```python
from build123d import *

# Parameters (mm, degrees)
SKETCH1_W              = 40
SKETCH1_H              = 60
BOSS_EXTRUDE1_DEPTH    = 10
M2_5_CLEARANCE_HOLE1_D = 2.9
CUT_EXTRUDE1_DEPTH     = 6.2
FILLET1_R              = 1.6
CHAMFER1_SIZE          = 1


with BuildPart() as part:
    # Sketch1 → Boss-Extrude1 (new body)
    with BuildSketch(Plane(origin=(0, 0, 0), x_dir=(1, 0, 0), z_dir=(0, 1, 0))):
        with Locations((-20, 0)):
            Rectangle(SKETCH1_W, SKETCH1_H)
    extrude(amount=BOSS_EXTRUDE1_DEPTH)

    # M2.5 Clearance Hole1 (through all)
    with Locations(Plane(origin=(0, 10, 0), x_dir=(1, 0, 0), z_dir=(0, 1, 0))):
        with Locations((-37.3, 26), (-37.3, 4), (-37.3, -18), (-31, -25.8), (-9, -25.8), (-2.7, -18), (-2.7, 4), (-2.7, 26)):
            Hole(M2_5_CLEARANCE_HOLE1_D / 2)

    # Sketch4 → Cut-Extrude1 (cut)
    with BuildSketch(Plane(origin=(0, 10, 0), x_dir=(1, 0, 0), z_dir=(0, 1, 0))):
        Polygon((-34.6, 30), (-34.6, -19), (-30, -19), (-30, -23), (-10, -23), (-10, -19), (-5.4, -19), (-5.4, 30), align=None)
    extrude(amount=-CUT_EXTRUDE1_DEPTH, mode=Mode.SUBTRACT)

    # Fillet1
    fillet1_edges = [part.edges().sort_by_distance(p)[0] for p in [
        (-10, 6.9, 23),
        (-30, 6.9, 23),
        (-30, 6.9, 19),
        (-34.6, 6.9, 19),
        (-5.4, 6.9, 19),
        (-10, 6.9, 19),
    ]]
    fillet(fillet1_edges, radius=FILLET1_R)

    # Chamfer1
    chamfer1_edges = [part.edges().sort_by_distance(p)[0] for p in [
        (-40, 5, -30),
        (0, 5, -30),
        (0, 5, 30),
        (-40, 5, 30),
    ]]
    chamfer(chamfer1_edges, length=CHAMFER1_SIZE)


solid = part.part
```
Geometry check sheet. Reference: the model listing, model coordinates, mm. A direction names the side the tool comes from. Round coordinates to 2 decimals unless told otherwise and drop trailing zeros. Order: outer loops, then holes, each group sorted by start corner. A loop starts at its lowest first (then second) coordinate and runs counter-clockwise, first axis right, second up. Notation, with made-up numbers: (-25.75, -38.75) - (-18.75, -38.75) arc R32 ccw to (-18.75, 0.25) - close; hole circle Ø11 at (-18.75, -4). An arc over 180 degrees is marked (long way). Use a Markdown table: item, result. Add a question column.
1) Mould release check, pull along X, two halves, no side actions. Record for faces 1 (the flat face through (-40, 5, 0)), 2 (the cylindrical face through (-7.93, 4.93, 24.82)), 3 (the cylindrical face through (-2.386, 4.93, 19.416)), 4 (the flat face through (-35, 10, 9)): released by +X, released by -X, zero draft, split by the parting line, or undercut.
2) Set-up check for faces 5 (the cylindrical face through (-30.48, 6.86, 19.46)), 6 (the cylindrical face through (-36.15, 4.93, -25.12)): record each of +Z, -Z, +X, -X, +Y, -Y from which the full face is reachable in a straight line by a thin tool's end or side.
3) Section check B-B (z = 25.8). Record the cut outline in (x, y), then the cut area to 3 significant figures.
4) Section check A-A (x = -2.7). Record the cut outline in (y, z), then the cut area to 3 significant figures.
5) Gauge pin test, flat ends, axial feed: P1, Ø6, axis at x = -25.5, z = -10, coming from the +Y side; P2, Ø5, axis at x = -18.5, y = 8.5, coming from the -Z side. Record the tip position at first contact, or that the pin passes through.
6) Section check C-C (y = 2). Count the separate pieces of the cut face and the enclosed holes in it, then the cut area to 3 significant figures.
7) Thickness scan on line 1 along Z through (x, y) = (-2.7, 3.5); line 2 along X through (y, z) = (6.25, 25.8); line 3 along X through (y, z) = (2.25, -26). Record the ranges inside material, lowest first.
Established:
| question | item | result |
|---|---|---|
| 1 | face 1 | released by -X |
| 1 | face 2 | undercut |
| 1 | face 3 | undercut |
| 1 | face 4 | zero draft |
| 2 | face 5 | -Z, +Y |
| 2 | face 6 | +Y, -Y |
| 3 | outline | (-40, 0) - (-32.45, 0) - (-32.45, 10) - (-40, 10) - close; (-29.55, 0) - (-10.45, 0) - (-10.45, 10) - (-29.55, 10) - close; (-7.55, 0) - (0, 0) - (0, 10) - (-7.55, 10) - close |
| 3 | area | 342 mm2 |
| 4 | outline | (0, -30) - (10, -30) - (10, -27.45) - (0, -27.45) - close; (0, -24.55) - (10, -24.55) - (10, -5.45) - (0, -5.45) - close; (0, -2.55) - (10, -2.55) - (10, 16.55) - (0, 16.55) - close; (0, 19.45) - (10, 19.45) - (10, 30) - (0, 30) - close |
| 4 | area | 513 mm2 |
| 5 | P1 | y = 3.8 |
| 5 | P2 | z = 23 |
| 6 | separate pieces | 1 |
| 6 | enclosed holes | 8 |
| 6 | area | 2,350 mm2 |
| 7 | line 1 | -30 to -27.45, -24.55 to -5.45, -2.55 to 16.55, 19.45 to 30 |
| 7 | line 2 | -40 to -32.45, -29.55 to -10.45, -7.55 to 0 |
| 7 | line 3 | -40 to -38.75, -35.85 to -4.15, -1.25 to 0 |
